Autodesk Inventor part; units mm, degrees
ref_plane "YZ Plane" through (0, 0, 0) normal (1, 0, 0) x (0, 1, 0)
ref_plane "XZ Plane" through (0, 0, 0) normal (0, 1, 0) x (-1, 0, 0)
ref_plane "XY Plane" through (0, 0, 0) normal (0, 0, 1) x (1, 0, 0)
sketch "SketchCircles" plane through (0, 0, 0) normal (0, 1, 0) x (-1, 0, 0)
  circle A0 centre (0, 0) radius 12.7
  circle A1 centre (0, 0) radius 6.35
  circle A2 centre (0, 0) radius 17.4625
  dimension "d0" = 25.4
  dimension "d1" = 12.7
  dimension "d2" = 34.925
extrude "Extrusion100" add sketch "SketchCircles" along normal blind 6.35 contours A0 | A1 | A2
sketch "SketchLines" plane through (0, 0, 0) normal (0, -1, 0) x (1, 0, 0)
  line L0 (-17.7365, 0) -> (17.5532, 0)
  line L1 (-0.0917, 17.7823) -> (-0.0917, -17.324)
  point P0 (0, 0)
hole "Hole1" at (0, 0, 0) direction (0, 1, 0) diameter 25.4 depth 3.175
sketch "Sketch3" plane through (0, 3.175, 0) normal (0, -1, 0) x (1, 0, 0)
  circle A0 centre (0, 0) radius 6.35
  dimension "d12" = 12.7
extrude "Extrusion2" add sketch "Sketch3" along normal blind 3.175
chamfer "Chamfer1" distance 1.397 angle 45 1 edges at (0, 0, 12.7)
chamfer "Chamfer2" distance 1.397 angle 45 1 edges at (-6.35, 0, 0)
sketch "Sketch4" plane through (0, 6.35, 0) normal (0, 1, 0) x (1, 0, 0)
  circle A0 centre (0, 0) radius 3.9688
  dimension "d21" = 7.9375
hole "Hole2" at (0, 6.35, 0) direction (0, -1, 0) diameter 6.35 depth 12.7
properties part number "tiedown-hook-mount"
Verification items for the finished model (mm, model axes). A direction names the side the tool comes from. Give positions to 0.01 mm unless a question says otherwise; leave off trailing zeros. Loops run counter-clockwise (first coordinate to the right, second up) from the corner with the lowest first, then second, coordinate; pieces in that order, holes last.
1. Section check D-D, the plane x = -14.5. Enter the section's corners in (y, z).
2. Thickness scan on line 1 (X direction, y = 0.75, z = 1.5); line 2 (Y direction, x = 4.5, z = -6) (3 decimals); line 3 (Z direction, x = -10, y = 3). Record the ranges inside material, lowest first.
3. Mould release check, pull along Z, two halves, no side actions. Record for faces 1 (the flat face through (-6, 3.175, -3)), 2 (the flat face through (3.2, 0, -1)), 3 (the cylindrical face through (13.858, 3.131, 10.626)): released by +Z, released by -Z, zero draft, split by the parting line, or undercut.
4. Go/stop test with flat-tipped pins: pin 1 Ø1.5 at (y, z) = (3, -11.5) entering from +X; pin 2 Ø6 at (x, z) = (-9.5, 0.5) entering from -Y (3 decimals); pin 3 Ø15 at (x, z) = (0, 0) entering from +Y; pin 4 Ø1.5 at (y, z) = (3, -2.5) entering from +X. Record where each tip stops, or that it passes through.
5. Set-up check for faces 4 (the cylindrical face through (12.4, 2.3, 2.75)), 5 (the cylindrical face through (3.1, 3.13, -0.69)): record each of +Z, -Z, +X, -X, +Y, -Y from which the full face is reachable in a straight line by a thin tool's end or side.
Geometry says:
1. outline: (0, -9.73) - (6.35, -9.73) - (6.35, 9.73) - (0, 9.73) - close
2. line 1: x = -17.4 to -13.26, -5.5 to -2.8, 2.8 to 5.5, 13.26 to 17.4
2. line 2: y = 3.175 to 6.35
2. line 3: z = -14.32 to -7.83, 7.83 to 14.32
3. face 1: undercut
3. face 2: zero draft
3. face 3: split by the parting line
4. pin 1: stops at x = 13.76
4. pin 2: stops at y = 3.175
4. pin 3: stops at y = 6.35
4. pin 4: stops at x = 17.37
5. face 4: -Y
5. face 5: +Y, -Y
